Work out the finished part from the listing and answer in its coordinate system (mm). Face numbers are marked on the shaded views. A direction names the side the tool comes from. Coordinates: 2 decimals unless noted, no trailing zeros. Order: outer loops, then holes, each group sorted by start corner. A loop starts at its lowest first (then second) coordinate and runs counter-clockwise, first axis right, second up. Notation, with made-up numbers: (-35, 33.25) -> (-22, 33.25) arc R19 ccw to (-22, 67.25) -> close; hole circle Ø9 at (11, 71.25). An arc over 180 degrees is marked (long way). Write item = value, one per line. Start each with the question number.
Q1. The part is cut by section D-D, the plane y = 13.5. Determine the outline of the cut face in (x, z).
Q2. The part is cut by section C-C, the plane x = 12.5. Determine the outline of the cut face in (y, z), plus the area to 3 significant figures.
Q3. Flat-ended cylindrical pins translate along their axes: pin 1 (1.9 mm diameter, centred on x = 21.5, y = 17.83, fed in from +Z); pin 2 (2 mm diameter, centred on x = 9, y = 16, fed in from +Z). Find the tip coordinate at first contact, or state that the pin passes through.
Q4. For a pull along X with two mould halves and no side action, classify the marked faces 3, 4 and 5 as +X half, -X half, draft (parallel to the pull), parting line (faces both ways), or undercut.
Q5. Straight lines are drawn through the part: L1, parallel to Y at x = 3.5, z = 0.45; L2, parallel to X at y = 7.5, z = 3; L3, parallel to Z at x = 22, y = 6.75. For each, find the intervals that lie inside material, in ascending order. Write a range as from..to.
Q6. The part is cut by section A-A, the plane x = 21.5. Determine the outline of the cut face in (y, z), plus the area to 3 significant figures.
Q7. The part is cut by section B-B, the plane z = 9.5. Determine the outline of the cut face in (x, y), plus the area to 3 significant figures.
Q8. Which of the six approach directions +Z, -Z, +X, -X, +Y, -Y give full straight-line access (tool end or side, diameter ignored) to the marked faces 1 and 2?
```python
from build123d import *

# Parameters (mm, degrees)
SKETCH_W      = 25
SKETCH_H      = 25
SKETCH_R      = 6
PAD_DEPTH     = 1.5
PAD001_DEPTH  = 20
SKETCH002_R   = 1.2
HOLE_DEPTH    = 25
CHAMFER_SIZE2 = 19
CHAMFER_SIZE  = 24


with BuildPart() as part:
    # Sketch → Pad (new body)
    with BuildSketch(Plane.XZ):
        with Locations((12.5, 12.5)):
            Rectangle(SKETCH_W, SKETCH_H)
        with Locations((12.5, 12.5)):
            Circle(SKETCH_R, mode=Mode.SUBTRACT)
    extrude(amount=PAD_DEPTH)

    # Sketch001 (on Face6 of Pad) → Pad001 (join)
    with BuildSketch(Plane(origin=(0, 0, 0), x_dir=(1, 0, 0), z_dir=(0, 1, 0))):
        Polygon((25, -25), (25, 0), (0, 0), (0, -25), (1, -25), (1, -1), (24, -1), (24, -25), align=None)
    extrude(amount=PAD001_DEPTH)

    # Sketch002 (on Face15 of Pad001) → Hole (cut)
    with BuildSketch(Plane(origin=(0, 0, 1), x_dir=(-1, 0, 0), z_dir=(0, 0, 1))):
        with Locations((-3.5, -17.826087)):
            Circle(SKETCH002_R)
        with Locations((-21.5, -17.826087)):
            Circle(SKETCH002_R)
        with Locations((-21.5, -2.173913)):
            Circle(SKETCH002_R)
        with Locations((-3.5, -2.173913)):
            Circle(SKETCH002_R)
    extrude(amount=-HOLE_DEPTH, mode=Mode.SUBTRACT)

    # Chamfer
    chamfer_edges = [part.edges().sort_by_distance(p)[0] for p in [
        (0.5, 20, 25),
        (24.5, 20, 25),
    ]]
    chamfer_side = part.faces().sort_by_distance((24.646447, 20, 12.5))[0]
    chamfer(chamfer_edges, length=CHAMFER_SIZE, length2=CHAMFER_SIZE2, reference=chamfer_side)


solid = part.part
```
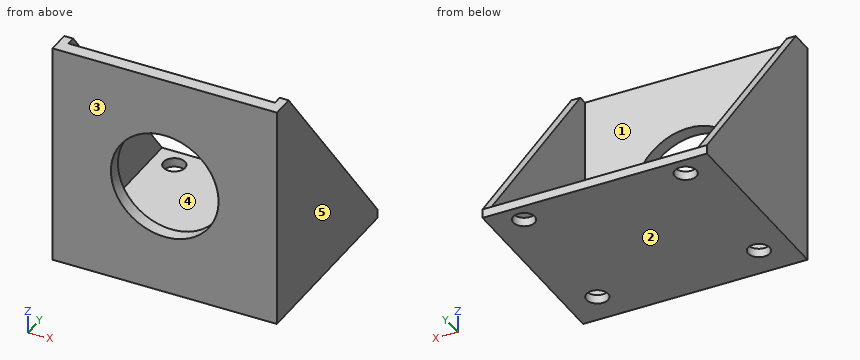
Model answer:
q1.outline = (0, 0) -> (25, 0) -> (25, 9.21) -> (24, 9.21) -> (24, 1) -> (1, 1) -> (1, 9.21) -> (0, 9.21) -> close
q2.outline = (-1.5, 0) -> (20, 0) -> (20, 1) -> (0, 1) -> (0, 6.5) -> (-1.5, 6.5) -> close; (-1.5, 18.5) -> (0, 18.5) -> (0, 25) -> (-1.5, 25) -> close
q2.area = 39.5 mm2
q3.pin_1 = through
q3.pin_2 = 1
q4.face_3 = draft
q4.face_4 = undercut
q4.face_5 = +X half
q5.L1 = -1.5..0.97, 3.37..16.63, 19.03..20
q5.L2 = 0..1, 24..25
q5.L3 = 0..1
q6.outline = (-1.5, 0) -> (0.97, 0) -> (0.97, 1) -> (0, 1) -> (0, 25) -> (-1.5, 25) -> close; (3.37, 0) -> (16.63, 0) -> (16.63, 1) -> (3.37, 1) -> close; (19.03, 0) -> (20, 0) -> (20, 1) -> (19.03, 1) -> close
q6.area = 52.7 mm2
q7.outline = (0, -1.5) -> (7.3, -1.5) -> (7.3, 0) -> (1, 0) -> (1, 13.27) -> (0, 13.27) -> close; (17.7, -1.5) -> (25, -1.5) -> (25, 13.27) -> (24, 13.27) -> (24, 0) -> (17.7, 0) -> close
q7.area = 48.5 mm2
q8.face_1 = +Z, +Y
q8.face_2 = -Z, +X, -X, +Y, -Y
